Geometry: final body of the model. Coordinates: model frame, mm. A direction names the side the tool comes from. Give positions to 0.01 mm unless a question says otherwise; leave off trailing zeros. Write each loop counter-clockwise with the first axis right and the second up, starting at its lowest first coordinate (ties: lowest second). Pieces come first, ordered by that corner, then holes. Notation, with made-up numbers: (81.5, 22.5) - (115.5, 22.5) arc R23 cw to (115.5, 46.5) - close; hole circle Ø10 at (88.5, 23.5). An arc over 180 degrees is marked (long way). One line per question, with ' | ' between items. Start each with the question number.
```python
from build123d import *

# Parameters (mm, degrees)
SKIZZE1_W                       = 15
SKIZZE1_H                       = 15
SKIZZE1_W_2                     = 13
SKIZZE1_H_2                     = 13
LINEAR_AUSTRAGEN_D_NN1_DEPTH    = 30
SKIZZE2_R                       = 1.75
SKIZZE2_R_2                     = 5
SCHNITT_LINEAR_AUSTRAGEN1_DEPTH = 17


with BuildPart() as part:
    # Skizze1 → Linear-Austragen-Dünn1 (new, symmetric)
    with BuildSketch(Plane.XY):
        Rectangle(SKIZZE1_W, SKIZZE1_H)
        Rectangle(SKIZZE1_W_2, SKIZZE1_H_2, mode=Mode.SUBTRACT)
    extrude(amount=LINEAR_AUSTRAGEN_D_NN1_DEPTH, both=True)

    # Skizze2 → Schnitt-Linear austragen1 (cut)
    with BuildSketch(Plane(origin=(0, 7.5, 0), x_dir=(1, 0, 0), z_dir=(0, 1, 0))):
        with Locations(Location((0, -22, 0), (0, 0, 270))):
            Circle(SKIZZE2_R)
        with Locations(Location((0, 8, 0), (0, 0, 270))):
            Circle(SKIZZE2_R)
        with Locations(Location((0, 20, 0), (0, 0, 270))):
            Circle(SKIZZE2_R_2)
    extrude(amount=-SCHNITT_LINEAR_AUSTRAGEN1_DEPTH, mode=Mode.SUBTRACT)


solid = part.part
```
1) Pull-direction query (Z, two-part tool) for faces 1 (the flat face through (-7.5, 0, 0)), 2 (the cylindrical face through (0.08, 7.01, 20.25)), 3 (the flat face through (-7, 0, 30)); classes: +Z half, -Z half, draft (parallel to the pull), parting line (faces both ways), or undercut.
2) Section D-D, the plane x = 0. Give the number of separate pieces and of enclosed holes in the cut face, plus the area to 3 significant figures.
3) Section B-B, the plane z = 22. Output: boundary loops of the cut face in (x, y).
4) First-contact query: pin 1 Ø4 at (x, z) = (0, -8) entering from -Y; pin 2 Ø2 at (x, z) = (0, 22) entering from +Y. Flat tips, straight axial feed; report the tip coordinate or a pass-through.
5) Reachability of faces 4 (the cylindrical face through (0, -7, -25)), 5 (the flat face through (0, 6.5, 0)) from +Z, -Z, +X, -X, +Y, -Y: full face, straight path, thin tool, end or side. Return the list, or none.
6) Line query: L1, parallel to X at y = 1.25, z = 20; L2, parallel to X at y = -7.2, z = 22. Output: solid intervals per line, ascending.
7) Section A-A, the plane y = 3.5. Output: boundary loops of the cut face in (x, z), plus the area to 3 significant figures.
Answer key:
1) face 1: draft | face 2: undercut | face 3: +Z half
2) separate pieces: 8 | enclosed holes: 0 | area: 86.0 mm^2
3) outline: (-7.5, -7.5) - (-1.75, -7.5) - (-1.75, -6.5) - (-6.5, -6.5) - (-6.5, 6.5) - (-1.75, 6.5) - (-1.75, 7.5) - (-7.5, 7.5) - close; (1.75, -7.5) - (7.5, -7.5) - (7.5, 7.5) - (1.75, 7.5) - (1.75, 6.5) - (6.5, 6.5) - (6.5, -6.5) - (1.75, -6.5) - close
4) pin 1: y = -7.5 | pin 2: through
5) face 4: +Y, -Y | face 5: +Z, -Z
6) L1: -7.5 to -6.5, 6.5 to 7.5 | L2: -7.5 to -1.75, 1.75 to 7.5
7) outline: (-7.5, -30) - (-6.5, -30) - (-6.5, 30) - (-7.5, 30) - close; (6.5, -30) - (7.5, -30) - (7.5, 30) - (6.5, 30) - close | area: 120 mm^2
